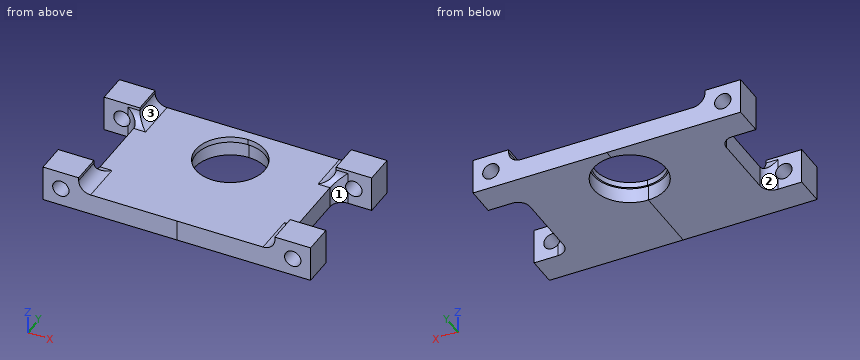
from build123d import *
from build123d.topology import SkipClean

# Parameters (mm, degrees)
BOSS_EXTRUDE1_DEPTH = 7
SKETCH2_W           = 12
SKETCH2_H           = 10
BOSS_EXTRUDE2_DEPTH = 12
FILLET1_R           = 4
FILLET2_R           = 4
SKETCH3_R           = 2.75
CUT_EXTRUDE1_DEPTH  = 104.653269711
SKETCH4_R           = 12.15
CUT_EXTRUDE2_DEPTH  = 5.1


with BuildPart() as part:
    # Sketch1 → Boss-Extrude1 (new body)
    with BuildSketch(Plane.XY):
        with BuildLine():
            Line((45.000001788, 50), (78.000001788, 50))
            Line((78.000001788, 50), (78.000001788, 0))
            Line((78.000001788, 0), (45.000001788, 0))
            Line((45.000001788, 0), (45.000001788, 23.4))
            ThreePointArc((45.000001788, 23.4), (56.600001788, 35), (45.000001788, 46.6))
            Line((45.000001788, 46.6), (45.000001788, 50))
        make_face()
    extrude(amount=BOSS_EXTRUDE1_DEPTH)

    # Sketch2 → Boss-Extrude2 (add)
    with BuildSketch(Plane(origin=(0, 0, 0), x_dir=(-1, 0, 0), z_dir=(0, 0, -1))):
        with Locations((-84.000001788, 45)):
            Rectangle(SKETCH2_W, SKETCH2_H)
        with Locations((-84.000001788, 5)):
            Rectangle(SKETCH2_W, SKETCH2_H)
    extrude(amount=-BOSS_EXTRUDE2_DEPTH)

    # Fillet1
    fillet1_edges = [part.edges().sort_by_distance(p)[0] for p in [
        (78.000001788, 40, 3.5),
        (78.000001788, 10, 3.5),
    ]]
    fillet(fillet1_edges, radius=FILLET1_R)

    # Fillet2
    fillet2_edges = [part.edges().sort_by_distance(p)[0] for p in [
        (78.000001788, 5, 7),
        (80.000001788, 10, 7),
        (78.000001788, 45, 7),
        (80.000001788, 40, 7),
    ]]
    fillet(fillet2_edges, radius=FILLET2_R - 0.0001)  # a hair under: the kernel refuses the full size

    # Sketch3 → Cut-Extrude1 (cut, through all)
    with BuildSketch(Plane(origin=(0, 50, 0), x_dir=(1, 0, 0), z_dir=(0, 1, 0))):
        with Locations(Location((84.000001788, -6, 0), (0, 0, 270))):
            Circle(SKETCH3_R)
    extrude(amount=-CUT_EXTRUDE1_DEPTH, mode=Mode.SUBTRACT)

    # Sketch4 → Cut-Extrude2 (cut)
    with BuildSketch(Plane(origin=(0, 0, 0), x_dir=(-1, 0, 0), z_dir=(0, 0, -1))):
        with Locations((-45.000001788, 35)):
            Circle(SKETCH4_R)
    extrude(amount=-CUT_EXTRUDE2_DEPTH, mode=Mode.SUBTRACT)

    # Mirror1: part across plane


with BuildPart() as part_1:
    with SkipClean():  # the faces are left unmerged after this step: merging them gives an invalid solid
        add(part.part)
        add(part.part.mirror(Plane(origin=(45.000001788, 23.4, 7), x_dir=(0, 0, 1), z_dir=(1, 0, 0))))


solid = part_1.part
Design review of the part built by this model. Coordinates are the model's own, in mm. Face numbers are marked on the shaded views. A direction names the side the tool comes from. Give positions to 0.01 mm unless a question says otherwise; leave off trailing zeros. Loops run counter-clockwise (first coordinate to the right, second up) from the corner with the lowest first, then second, coordinate; pieces in that order, holes last. Notation, with made-up numbers: M -5.5,83.5 L 25.5,83.5 A15 ccw 25.5,109.5 Z; hole C 49.5,38 d5. An arc over 180 degrees is marked long. Answer as a JSON object with one key per item and string values.
Item 1: Machinability: for the marked faces 1, 2 and 3, which of the approach directions +Z, -Z, +X, -X, +Y, -Y give a long, thin tool a straight path to every point of the face, cutting with its end or side? Answer none if there is none.
Output values:
{"face 1": "+Z, -Z, +X", "face 2": "+Z, -Z, -X", "face 3": "+Z, +Y, -Y"}
Item 2: We need section A-A (z = 6). Count the separate pieces of the cut face and the enclosed holes in it, and give its area (3 significant figures).
Output values:
{"separate pieces": "5", "enclosed holes": "1", "area": "3,150 mm2"}
Item 3: We need section D-D (y = 15.5). State the section outline as (x, z) points.
Output values:
{"outline": "M 12,0 L 78,0 L 78,7 L 12,7 Z"}
Item 4: We need section B-B (y = 25.5). State the section outline as (x, z) points, and give its area (3 significant figures).
Output values:
{"outline": "M 12,0 L 37.43,0 L 37.43,5.1 L 38.34,5.1 L 38.34,7 L 12,7 Z; M 51.66,5.1 L 52.57,5.1 L 52.57,0 L 78,0 L 78,7 L 51.66,7 Z", "area": "359 mm2"}
Item 5: Wall thickness on line 1 along X through (y, z) = (5.5, 6); line 2 along Z through (x, y) = (17.5, 23); line 3 along X through (y, z) = (42.5, 11): over which ranges is each line inside the solid? List them lowest first.
Output values:
{"line 1": "x = 0 to 3.25, 8.75 to 81.25, 86.75 to 90", "line 2": "z = 0 to 7", "line 3": "x = 0 to 12, 78 to 90"}
Item 6: We need section C-C (x = 39). State the section outline as (y, z) points, and give its area (3 significant figures).
Output values:
{"outline": "M 0,0 L 24.43,0 L 24.43,5.1 L 25.07,5.1 L 25.07,7 L 0,7 Z; M 44.93,5.1 L 45.57,5.1 L 45.57,0 L 50,0 L 50,7 L 44.93,7 Z", "area": "205 mm2"}
Item 7: For P1, Ø5.5, axis at y = 26, z = 3, coming from the -X side; P2, Ø1.5, axis at x = 61, y = 26.5, coming from the +Z side; P3, Ø4, axis at y = 37, z = 3, coming from the +X side, all flat-tipped, find the tip position at first contact; note any pin that passes through.
Output values:
{"P1": "stops at x = 12", "P2": "stops at z = 7", "P3": "stops at x = 79.35"}
